Work out the finished part from the listing and answer in its coordinate system (mm). Give positions to 0.01 mm unless a question says otherwise; leave off trailing zeros. Order: outer loops, then holes, each group sorted by start corner. A loop starts at its lowest first (then second) coordinate and runs counter-clockwise, first axis right, second up. Notation, with made-up numbers: (45, 10) -> (50, 10) arc R21 ccw to (50, 35) -> close; hole circle Ø4 at (2, 76). An arc over 180 degrees is marked (long way). Answer as CSV lines item,"result". Start each with the question number.
1. Flat-ended cylindrical pins translate along their axes: pin 1 (2.5 mm diameter, centred on x = -38.5, y = -2, fed in from +Z); pin 2 (2.5 mm diameter, centred on y = -1.5, z = 36, fed in from -X). Find the tip coordinate at first contact, or state that the pin passes through.
2. A cutting plane is placed at C-C (x = -15). Give the vertices of the cut face in (y, z), then the cut area to 3 significant figures.
3. A cutting plane is placed at B-B (z = 14). Give the vertices of the cut face in (x, y), then the cut area to 3 significant figures.
4. Find the intervals of material crossed by L1, parallel to X at y = -4.8, z = 13; L2, parallel to X at y = -3.95, z = 97; L3, parallel to X at y = -2.05, z = 73.5, in increasing order.
from build123d import *

# Parameters (mm, degrees)
F1_DEPTH = 5


with BuildPart() as f1:
    # F0 (on Front) → F1 (new body)
    with BuildSketch(Plane.XZ):
        Polygon((-40, 10), (-40, 0), (0, 0), (0, 70), (-40, 70), (-40, 60), (-35, 60), (-35, 50), (-40, 50), (-40, 40), (-35, 40), (-35, 30), (-40, 30), (-40, 20), (-35, 20), (-35, 10), align=None)
        Polygon((0, 70), (0, 0), (40, 0), (40, 10), (35, 10), (35, 20), (40, 20), (40, 30), (35, 30), (35, 40), (40, 40), (40, 50), (35, 50), (35, 60), (40, 60), (40, 70), align=None)
        Polygon((-40, 70), (0, 70), (-20, 106.853262), align=None)
        Polygon((20, 106.853262), (0, 70), (40, 70), align=None)
    extrude(amount=F1_DEPTH)


solid = f1.part
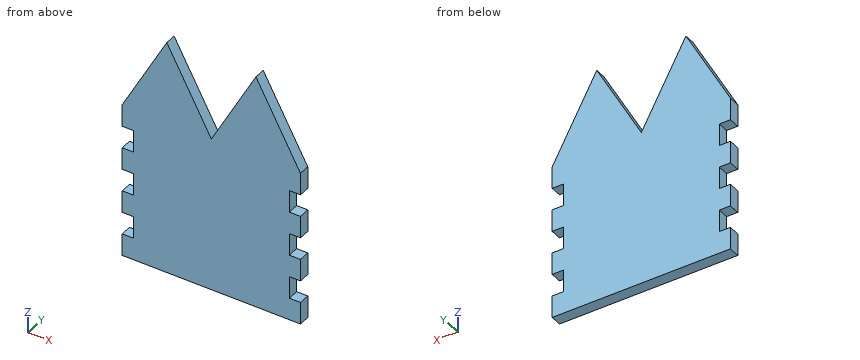
Answer sheet:
1,pin 1,"stops at z = 75.07"
1,pin 2,"stops at x = -35"
2,outline,"(-5, 0) -> (0, 0) -> (0, 97.64) -> (-5, 97.64) -> close"
2,area,"488 mm^2"
3,outline,"(-35, -5) -> (35, -5) -> (35, 0) -> (-35, 0) -> close"
3,area,"350 mm^2"
4,L1,"x = -35 to 35"
4,L2,"x = -25.35 to -14.65, 14.65 to 25.35"
4,L3,"x = -38.1 to -1.9, 1.9 to 38.1"
